```python
from build123d import *

# Parameters (mm, degrees)
SKETCH3_R      = 18.5
EXTRUDE1_DEPTH = 20
SKETCH4_R      = 14
EXTRUDE2_DEPTH = 14
SKETCH5_R      = 18.5
EXTRUDE3_DEPTH = 10


with BuildPart() as part:
    # Sketch2 → Revolve1 (revolve)
    with BuildSketch(Plane.XY, mode=Mode.PRIVATE) as revolve1_sk:
        Polygon((0, 0), (0, 120), (4, 120), (4, 140), (29, 140), (29, 130), (14, 130), (14, 115), (5, 115), (5, 0), align=None)
    revolve(revolve1_sk.sketch.rotate(Axis((-12, -9.379740318, 0), (0, 1, 0)), 90), axis=Axis((-12, -9.379740318, 0), (0, 1, 0)))

    # Sketch3 → Extrude1 (cut)
    with BuildSketch(Plane.XZ):
        with Locations((-12, 0)):
            Circle(SKETCH3_R)
    extrude(amount=-EXTRUDE1_DEPTH, mode=Mode.SUBTRACT)

    # Sketch4 → Extrude2 (cut)
    with BuildSketch(Plane.XZ.offset(-20)):
        with Locations(Location((-12, 0, 0), (0, 0, 270))):
            Circle(SKETCH4_R)
    extrude(amount=-EXTRUDE2_DEPTH, mode=Mode.SUBTRACT)

    # Sketch5 → Extrude3 (cut)
    with BuildSketch(Plane(origin=(0, 140, 0), x_dir=(1, 0, 0), z_dir=(0, 1, 0))):
        with Locations(Location((-12, 0, 0), (0, 0, 270))):
            Circle(SKETCH5_R)
    extrude(amount=-EXTRUDE3_DEPTH, mode=Mode.SUBTRACT)


solid = part.part
```
Source: CAD feature listing. Evaluate the final solid. Frame: model axes, mm. A direction names the side the tool comes from. Give positions to 0.01 mm unless a question says otherwise; leave off trailing zeros. Order: outer loops, then holes, each group sorted by start corner. A loop starts at its lowest first (then second) coordinate and runs counter-clockwise, first axis right, second up.
(1) Section query C-C (y = 100). Return the cut outline in (x, z).
(2) Material intervals for line 1 along X through (y, z) = (126, 0); line 2 along X through (y, z) = (53, 0); line 3 along Y through (x, z) = (9.5, -31.5), sorted ascending.
(3) Section query B-B (z = 0). Return the cut outline in (x, y), plus the area to 3 significant figures.
(4) Section query A-A (x = -12). Return the cut outline in (y, z).
(5) Contact query for flat-ended pins moving along their axis: P1, Ø10, axis at x = 6.5, y = 64, coming from the -Z side; P2, Ø12, axis at x = -33, z = -27, coming from the -Y side; P3, Ø1, axis at y = 32, z = -18, coming from the +X side; P4, Ø18.5, axis at x = -6, z = -2.5, coming from the +Y side. Output: stop coordinate, or through.
(6) Section query D-D (x = 19.5). Return the cut outline in (y, z), plus the area to 3 significant figures.
(7) Access query for faces 4 (the face through (-6.443, 135.07, 17.646)), 5 (the face through (13.38, 122.4, 5.64)), 6 (the face through (-3, 140, 18)). Directions: +Z, -Z, +X, -X, +Y, -Y. A direction counts if a zero-diameter tool reaches every point of the face in a straight line with its end or side. Return the directions, or none.
(8) Pull-direction query (X, two-part tool) for faces 1 (the face through (5, 115, -5)), 2 (the face through (-1.6, 34, 6.3)), 3 (the face through (28, 135, 9)); classes: +X half, -X half, draft (parallel to the pull), parting line (faces both ways), or undercut.
Outcome:
1. outline: circle Ø34 at (-12, 0); hole circle Ø24 at (-12, 0)
2. line 1: x = -38 to -28, 4 to 14
2. line 2: x = -29 to -24, 0 to 5
2. line 3: y = 130 to 140
3. outline: (-53, 130) - (-38, 130) - (-38, 115) - (-29, 115) - (-29, 20) - (-26, 20) - (-26, 34) - (-24, 34) - (-24, 120) - (-28, 120) - (-28, 130) - (-30.5, 130) - (-30.5, 140) - (-53, 140) - close; (0, 34) - (2, 34) - (2, 20) - (5, 20) - (5, 115) - (14, 115) - (14, 130) - (29, 130) - (29, 140) - (6.5, 140) - (6.5, 130) - (4, 130) - (4, 120) - (0, 120) - close
3. area: 1,680 mm2
4. outline: (20, -17) - (115, -17) - (115, -26) - (130, -26) - (130, -41) - (140, -41) - (140, -18.5) - (130, -18.5) - (130, -16) - (120, -16) - (120, -12) - (34, -12) - (34, -14) - (20, -14) - close; (20, 14) - (34, 14) - (34, 12) - (120, 12) - (120, 16) - (130, 16) - (130, 18.5) - (140, 18.5) - (140, 41) - (130, 41) - (130, 26) - (115, 26) - (115, 17) - (20, 17) - close
5. P1: stops at z = -10.33
5. P2: stops at y = 130
5. P3: passes through
5. P4: stops at y = 120
6. outline: (130, -26.24) - (140, -26.24) - (140, 26.24) - (130, 26.24) - close
6. area: 525 mm2
7. face 4: +Y
7. face 5: -Y
7. face 6: +Z, -Z, +X, -X, +Y
8. face 1: draft
8. face 2: undercut
8. face 3: parting line
